from build123d import *

# Parameters (mm, degrees)
F1_DEPTH = 3.175
F3_DEPTH = 9.144


with BuildPart() as f1:
    # F0 (on Front) → F1 (new body)
    with BuildSketch(Plane.XZ):
        Polygon((-42.153828, 7.319395), (-48.445281, 3.988625), (-42.153828, 1.768112), (-32.716647, 0), (-26.240151, -1.7477), (-17.573407, -5.396928), (-17.31674, -5.396928), (-15.692713, -7.484026), (-15.692713, -10.074626), (0, -10.074626), (10.953447, -5.396928), (22.796184, 1.768112), (25.94191, 5.283925), (28.717551, 9.724951), (31.86328, 13.425807), (34.638923, 19.532219), (34.638923, 21.752732), (34.638923, 23.788201), (31.86328, 23.788201), (28.717551, 21.752732), (25.94191, 19.532219), (22.796184, 18.051876), (18.910285, 16.571533), (10.953447, 16.571533), (-1.629462, 16.571533), (-15.692713, 14.906148), (-24.389723, 13.425807), (-30.681178, 11.760422), (-36.417503, 9.724951), align=None)
    extrude(amount=F1_DEPTH)

    # F2 (on Front) → F3 (cut)
    with BuildSketch(Plane.XZ):
        with BuildLine():
            Line((23.116694, 10.099179), (-23.068567, 1.39489))
            ThreePointArc((-23.068567, 1.39489), (-24.319738, -0.537971), (-22.327608, -1.69244))
            Line((-22.327608, -1.69244), (23.825702, 7.004356))
            ThreePointArc((23.825702, 7.004356), (25.080102, 8.920359), (23.116694, 10.099179))
        make_face()
    extrude(amount=F3_DEPTH, mode=Mode.SUBTRACT)


solid = f1.part
Could you check a few things on this model? Use its own coordinates, in mm. A direction names the side the tool comes from. Give positions to 0.01 mm unless a question says otherwise; leave off trailing zeros. Loops run counter-clockwise (first coordinate to the right, second up) from the corner with the lowest first, then second, coordinate; pieces in that order, holes last. Notation, with made-up numbers: (-10.75, 54.25) -> (26.25, 54.25) arc R5 ccw to (26.25, 63.25) -> close; hole circle Ø8 at (67.5, -34). An arc over 180 degrees is marked (long way). Return JSON: item names as keys, results as strings.
Item 1: If we section it at C-C on z = 2.5: List the corners of the cut face in (x, y) for me (3 decimals).
Geometry results:
{"outline": "(-44.228, -3.175) -> (-17.205, -3.175) -> (-17.205, 0) -> (-44.228, 0) -> close; (-0.079, -3.175) -> (23.451, -3.175) -> (23.451, 0) -> (-0.079, 0) -> close"}
Item 2: If we section it at D-D on z = -3.5: List the corners of the cut face in (x, y) for me (3 decimals).
Geometry results:
{"outline": "(-22.079, -3.175) -> (14.089, -3.175) -> (14.089, 0) -> (-22.079, 0) -> close"}
Item 3: Which directions (+Z, -Z, +X, -X, +Y, -Y) give clear straight access to the entire face, cutting with the end or side of a thin tool? Please do faces 1 (the flat face through (-29.524, -1.565, -0.862)), 2 (the flat face through (9, -2, 16.572)).
Geometry results:
{"face 1": "-Z, -X, +Y, -Y", "face 2": "+Z, -X, +Y, -Y"}
Item 4: I need wall thicknesses on L1, parallel to Z at x = -9.5, y = -2; L2, parallel to Z at x = -21, y = -0.75; L3, parallel to Z at x = 29, y = -1.6. Which ranges of each line are inside material? Lowest first, please. Write a range as from..to.
Geometry results:
{"L1": "z = -10.07..0.72, 3.95..15.64", "L2": "z = -3.95..-1.44, 1.78..14", "L3": "z = 10.06..21.94"}
Item 5: If we section it at B-B on x = 14: List the corners of the cut face in (y, z) for me (3 decimals).
Geometry results:
{"outline": "(-3.175, -3.554) -> (0, -3.554) -> (0, 5.153) -> (-3.175, 5.153) -> close; (-3.175, 8.381) -> (0, 8.381) -> (0, 16.572) -> (-3.175, 16.572) -> close"}
Item 6: We'd pull the mould along Z, two halves only. Please class faces 3 (the flat face through (16.792, -1.565, -1.865)), 4 (the cylindrical face through (-24.33, -1.57, -0.5)), 5 (the flat face through (-33.509, -1.565, 10.757)): +Z half, -Z half, draft (parallel to the pull), parting line (faces both ways), or undercut.
Geometry results:
{"face 3": "-Z half", "face 4": "undercut", "face 5": "+Z half"}
Item 7: I'm going to push a flat-ended pin straight in: pin 1 (1 mm diameter, centred on x = -12.5, z = 17.5, fed in from -Y). Where does the tip first touch, or does it pass through?
Geometry results:
{"pin 1": "passes through"}
